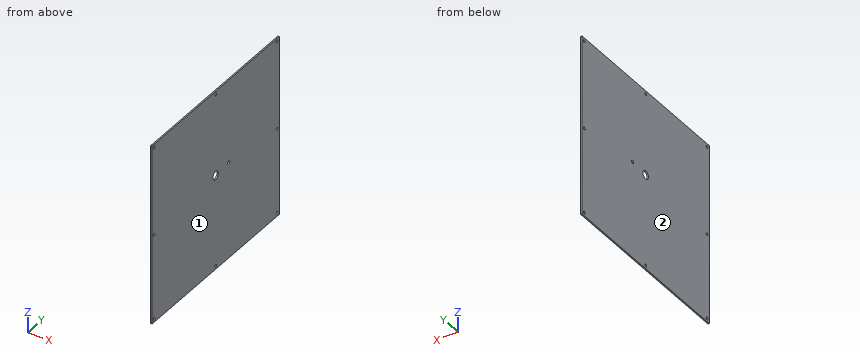
from build123d import *

# Parameters (mm, degrees)
SKETCH1_W                  = 368.3
SKETCH1_H                  = 368.3
BOSS_EXTRUDE1_DEPTH        = 2.54
F_6_0_204_DIAMETER_HOLE1_D = 5.1816
SKETCH3_W                  = 19.05
SKETCH3_H                  = 368.3
CUT_EXTRUDE1_DEPTH         = 2.54
SKETCH4_R                  = 8
CUT_EXTRUDE2_DEPTH         = 3.54
SKETCH5_R                  = 3.175
CUT_EXTRUDE3_DEPTH         = 2.54


with BuildPart() as part:
    # Sketch1 → Boss-Extrude1 (new body)
    with BuildSketch(Plane(origin=(0, 0, 0), x_dir=(0, 0, -1), z_dir=(1, 0, 0))):
        with Locations((184.15, 184.15)):
            Rectangle(SKETCH1_W, SKETCH1_H)
    extrude(amount=BOSS_EXTRUDE1_DEPTH)

    # #6 (0.204) Diameter Hole1 (through all)
    with Locations(Plane(origin=(2.54, 361.95, -361.95), x_dir=(0, 0, 1), z_dir=(1, 0, 0))):
        with Locations((0, 0), (0, 355.6), (336.55, 355.6), (336.55, 0), (336.55, 177.8), (0, 177.8), (165.1, 355.6), (165.1, 0)):
            Hole(F_6_0_204_DIAMETER_HOLE1_D / 2)

    # Sketch3 → Cut-Extrude1 (cut)
    with BuildSketch(Plane.ZY):
        with Locations((-9.525, 184.15)):
            Rectangle(SKETCH3_W, SKETCH3_H)
    extrude(amount=-CUT_EXTRUDE1_DEPTH, mode=Mode.SUBTRACT)

    # Sketch4 → Cut-Extrude2 (cut, through all)
    with BuildSketch(Plane.ZY):
        with Locations((-184.15, 184.15)):
            Circle(SKETCH4_R)
    extrude(amount=-CUT_EXTRUDE2_DEPTH, mode=Mode.SUBTRACT)

    # Sketch5 → Cut-Extrude3 (cut)
    with BuildSketch(Plane.ZY):
        with Locations((-180.737580342, 221.844041513)):
            Circle(SKETCH5_R)
    extrude(amount=-CUT_EXTRUDE3_DEPTH, mode=Mode.SUBTRACT)


solid = part.part
Can you work these out from the model? Positions are in its coordinate system, mm. Face numbers are marked on the shaded views. Coordinates: 2 decimals unless noted, no trailing zeros. Answer as a JSON object with one key per item and string values. Group by question number.
Item 1: If I drill on L1, parallel to Y at x = 0.8, z = -25.4; L2, parallel to Z at x = 1.95, y = 6.35; L3, parallel to Y at x = 1.5, z = -196.85, over which ranges is the centre line in solid material (lowest first)? Write a range as from..to.
Item 2: For pin 1 (3 mm diameter, centred on y = 361.95, z = -361.95, fed in from -X), with a flat end and sliding along its axis, tell me the tip position at first contact or that it passes through.
Item 3: If we mould it in two halves opening along X, with no side actions, what happens to the marked faces 1 and 2? For each: released by +X, released by -X, zero draft, split by the parting line, or undercut.
Returned:
{
 "1": {"L1": "y = 0..3.76, 8.94..181.56, 186.74..359.36, 364.54..368.3", "L2": "z = -368.3..-364.54, -359.36..-199.44, -194.26..-27.99, -22.81..-19.05", "L3": "y = 0..3.76, 8.94..359.36, 364.54..368.3"},
 "2": {"pin 1": "passes through"},
 "3": {"face 1": "released by +X", "face 2": "released by -X"}
}
